Design review of the part built by this model. Coordinates are the model's own, in mm. Round coordinates to 2 decimals unless told otherwise and drop trailing zeros. Use a Markdown table: item, result. Add a question column.
from build123d import *

# Parameters (mm, degrees)
F0_W      = 304.8
F0_H      = 38.1
F1_DEPTH  = 19.05
F2_R      = 11.1125
F3_DEPTH  = 12.7
F4_R      = 3.175
F5_DEPTH  = 19.051
F6_R      = 3.175
F7_DEPTH  = 19.051
F8_R      = 0.79375
F9_DEPTH  = 19.051
F10_W     = 3.175
F10_H     = 1.5875
F11_DEPTH = 38.101
F12_R     = 2.286
F13_DEPTH = 6.35


with BuildPart() as f1:
    # F0 (on Top) → F1 (new body)
    with BuildSketch(Plane.XY):
        with Locations((84.480461, 0)):
            Rectangle(F0_W, F0_H)
    extrude(amount=F1_DEPTH)

    # F2 (on face) → F3 (cut)
    with BuildSketch(Plane.XY.offset(19.05)):
        with Locations((135.280461, 0)):
            Circle(F2_R)
    extrude(amount=-F3_DEPTH, mode=Mode.SUBTRACT)

    # F4 (on face) → F5 (cut, through all)
    with BuildSketch(Plane.XY.offset(19.05)):
        with Locations((-58.394539, -3.175)):
            Circle(F4_R)
    extrude(amount=-F5_DEPTH, mode=Mode.SUBTRACT)

    # F6 (on face) → F7 (cut, through all)
    with BuildSketch(Plane.XY.offset(19.05)):
        with Locations((-24.612539, -9.525)):
            Circle(F6_R)
        with Locations((-24.612539, 9.525)):
            Circle(F6_R)
    extrude(amount=-F7_DEPTH, mode=Mode.SUBTRACT)

    # F8 (on face) → F9 (cut, through all)
    with BuildSketch(Plane.XY.offset(19.05)):
        with Locations((230.530461, 9.525)):
            Circle(F8_R)
        with Locations((230.530461, 0)):
            Circle(F8_R)
        with Locations((230.530461, -9.525)):
            Circle(F8_R)
    extrude(amount=-F9_DEPTH, mode=Mode.SUBTRACT)

    # F10 (on face) → F11 (cut, through all)
    with BuildSketch(Plane.XZ.offset(19.05)):
        with Locations((-9.182039, 18.25625)):
            Rectangle(F10_W, F10_H)
        with Locations((216.242961, 18.25625)):
            Rectangle(F10_W, F10_H)
    extrude(amount=-F11_DEPTH, mode=Mode.SUBTRACT)

    # F12 (on face) → F13 (cut, through all)
    with BuildSketch(Plane.XY.offset(6.35)):
        with Locations((135.280461, 0)):
            Circle(F12_R)
    extrude(amount=-F13_DEPTH, mode=Mode.SUBTRACT)


solid = f1.part
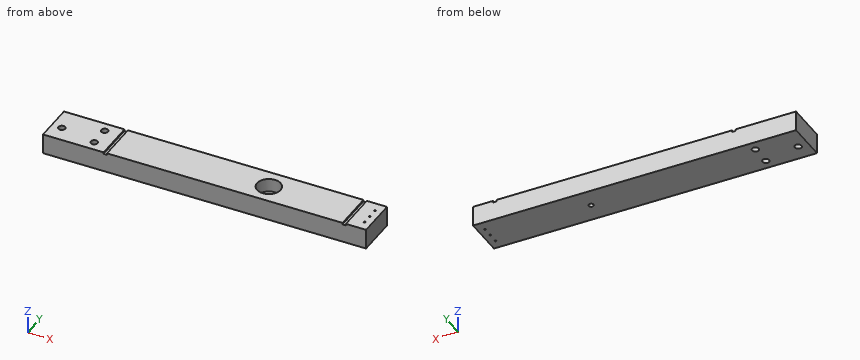
1. To check wall thickness, follow probe 1 along X at (y, z) = (-4.5, 9.25); probe 2 along X at (y, z) = (1, 9.25); probe 3 along Y at (x, z) = (131, 9.75). State the ranges of each line that lie inside material, in increasing order. Write a range as from..to.
2. Consider section A-A on z = 14.75. Give the number of separate pieces and of enclosed holes in the cut face, plus the area to 3 significant figures.
3. Insertion check: P1, Ø7.5, axis at x = 135.28, y = 0, coming from the +Z side; P2, Ø2.5, axis at x = -9, y = -6.5, coming from the +Z side. Each pin has a flat end and moves straight along its axis. Give the tip position at first contact, or say it passes through.
Verdict:
| question | item | result |
|---|---|---|
| 1 | probe 1 | x = -67.92..-61.28, -55.51..125.12, 145.44..236.88 |
| 1 | probe 2 | x = -67.92..124.21, 146.35..236.88 |
| 1 | probe 3 | y = -19.05..-10.26, 10.26..19.05 |
| 2 | separate pieces | 1 |
| 2 | enclosed holes | 7 |
| 2 | area | 11,100 mm² |
| 3 | P1 | stops at z = 6.35 |
| 3 | P2 | stops at z = 17.46 |
